Answer from the drawing. Dimensions are ordinates in mm from the lowest x, y and z of the part. Coordinates: 2 decimals unless noted, no trailing zeros. Loops run counter-clockwise (first coordinate to the right, second up) from the corner with the lowest first, then second, coordinate; pieces in that order, holes last. Notation, with made-up numbers: (4.5, 13) - (47.5, 13) arc R28 ccw to (47.5, 46) - close; hole circle Ø6 at (6.25, -35). An arc over 180 degrees is marked (long way). Use one line per item in the form item = value. Start each with the question number.
1) Consider line 1 (X direction, y = 1.9, z = 40); line 2 (X direction, y = 1.9, z = 64). Determine where each line is inside the solid, lowest interval first.
2) A cutting plane is placed at A-A (z = 40). Give the vertices of the cut face in (x, y), and give its area (3 significant figures).
3) A cutting plane is placed at B-B (x = 40). Give the vertices of the cut face in (y, z).
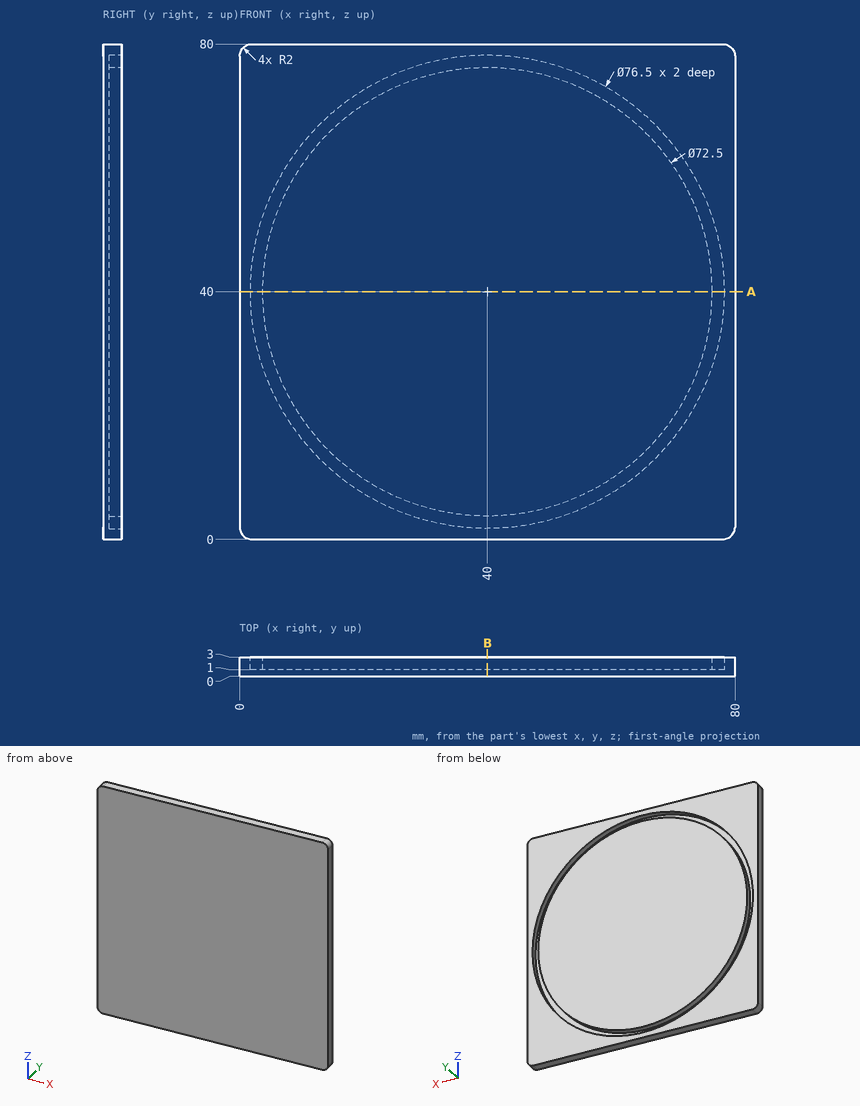
Found:
q1.line_1 = 0 to 1.75, 3.75 to 76.25, 78.25 to 80
q1.line_2 = 0 to 10.22, 12.83 to 67.17, 69.78 to 80
q2.outline = (0, 0) - (80, 0) - (80, 3) - (78.25, 3) - (78.25, 1) - (76.25, 1) - (76.25, 3) - (3.75, 3) - (3.75, 1) - (1.75, 1) - (1.75, 3) - (0, 3) - close
q2.area = 232 mm^2
q3.outline = (0, 0) - (3, 0) - (3, 1.75) - (1, 1.75) - (1, 3.75) - (3, 3.75) - (3, 76.25) - (1, 76.25) - (1, 78.25) - (3, 78.25) - (3, 80) - (0, 80) - close
